Build history of the part. All positions in model axes, mm. Give positions to 0.01 mm unless a question says otherwise; leave off trailing zeros. Loops run counter-clockwise (first coordinate to the right, second up) from the corner with the lowest first, then second, coordinate; pieces in that order, holes last. Notation, with made-up numbers: (-40, 72) -> (-7, 72) arc R10 cw to (-7, 85) -> close; hole circle Ø8 at (-27.75, 87.25). An arc over 180 degrees is marked (long way). One line per question, with ' | ' between items. Start each with the question number.
(1) Flat gauge pins, fed straight in: pin 1 Ø3 at (y, z) = (4, -6) entering from -X; pin 2 Ø2 at (y, z) = (2, -8.5) entering from +X; pin 3 Ø2 at (y, z) = (5.5, 14.5) entering from +X. Where does each tip first touch, or does it go through?
(2) Slice it at A-A, the plane y = 1.25. Give the number of separate pieces and of enclosed holes in the cut face, then the cut area to 3 significant figures.
(3) Drill centre lines: L1, parallel to X at y = 3, z = 0; L2, parallel to X at y = 2.75, z = 5.5; L3, parallel to Z at x = -135, y = 5. Where is each one in solid material? Low to high. Write a range as from..to.
(4) Slice it at B-B, the plane z = -2.5. Write the cut outline in (x, y), then the cut area to 3 significant figures.
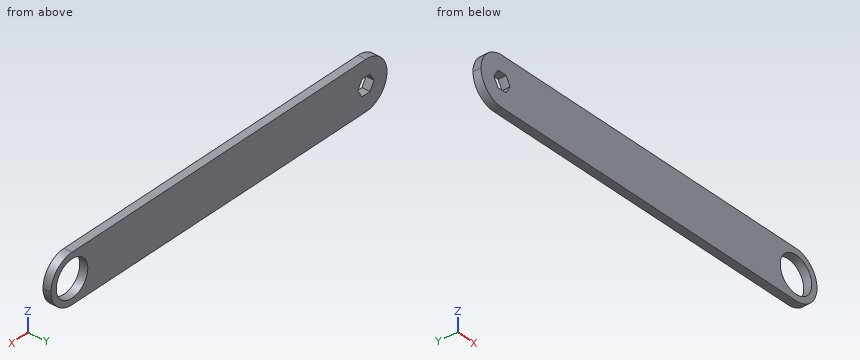
```python
from build123d import *

# Parameters (mm, degrees)
SKETCH1_W           = 304.8
SKETCH1_H           = 38.1
BOSS_EXTRUDE1_DEPTH = 6.35
SKETCH2_R           = 14.3002
CUT_EXTRUDE1_DEPTH  = 6.35
CUT_EXTRUDE5_DEPTH  = 6.35
FILLET3_R           = 19.05


with BuildPart() as part:
    # Sketch1 → Boss-Extrude1 (new body)
    with BuildSketch(Plane(origin=(0, 0, 0), x_dir=(1, 0, 0), z_dir=(0, 1, 0))):
        Rectangle(SKETCH1_W, SKETCH1_H)
    extrude(amount=BOSS_EXTRUDE1_DEPTH)

    # Sketch2 → Cut-Extrude1 (cut)
    with BuildSketch(Plane(origin=(0, 6.35, 0), x_dir=(1, 0, 0), z_dir=(0, 1, 0))):
        with Locations(Location((133.35, 0, 0), (0, 0, 270))):
            Circle(SKETCH2_R)
    extrude(amount=-CUT_EXTRUDE1_DEPTH, mode=Mode.SUBTRACT)

    # Sketch8 → Cut-Extrude5 (cut)
    with BuildSketch(Plane(origin=(0, 6.35, 0), x_dir=(1, 0, 0), z_dir=(0, 1, 0))):
        Polygon((-129.683825791, 6.35), (-137.016174209, 6.35), (-140.682348419, 0), (-137.016174209, -6.35), (-129.683825791, -6.35), (-126.017651581, 0), align=None)
    extrude(amount=-CUT_EXTRUDE5_DEPTH, mode=Mode.SUBTRACT)

    # Fillet3
    fillet3_edges = [part.edges().sort_by_distance(p)[0] for p in [
        (152.4, 3.175, 19.05),
        (152.4, 3.175, -19.05),
        (-152.4, 3.175, 19.05),
        (-152.4, 3.175, -19.05),
    ]]
    fillet(fillet3_edges, radius=FILLET3_R - 0.0001)  # a hair under: the kernel refuses the full size


solid = part.part
```
Final values:
1) pin 1: x = -151.86 | pin 2: x = 150.86 | pin 3: x = 146.79
2) separate pieces: 1 | enclosed holes: 2 | area: 10,500 mm2
3) L1: -152.4..-140.68, -126.02..119.05, 147.65..152.4 | L2: -151.59..-137.51, -129.19..120.15, 146.55..151.59 | L3: -18.98..-6.35, 6.35..18.98
4) outline: (-152.24, 0) -> (-139.24, 0) -> (-139.24, 6.35) -> (-152.24, 6.35) -> close; (-127.46, 0) -> (119.27, 0) -> (119.27, 6.35) -> (-127.46, 6.35) -> close; (147.43, 0) -> (152.24, 0) -> (152.24, 6.35) -> (147.43, 6.35) -> close | area: 1,680 mm2
